Geometry: final body of the model. Coordinates: model frame, mm. A direction names the side the tool comes from. Give positions to 0.01 mm unless a question says otherwise; leave off trailing zeros. Write each loop counter-clockwise with the first axis right and the second up, starting at its lowest first coordinate (ties: lowest second). Pieces come first, ordered by that corner, then holes.
Q1. Cut plane A-A on y = 17.78. Return the cut outline in (x, z) (1 decimal), plus the area to 3 significant figures.
Q2. Reachability of faces 1 (the face through (-9.755, 36.535, 5.017)), 2 (the face through (-1.588, -1, 25)), 3 (the face through (1.588, 1, 25)) from +Z, -Z, +X, -X, +Y, -Y: full face, straight path, thin tool, end or side. Return the list, or none.
Q3. Cut plane C-C on y = -4.5. Return the cut outline in (x, z), plus the area to 3 significant figures.
Q4. Pin query (flat end, axial travel): pin 1 (6.5 mm diameter, centred on x = -9.5, z = 17.5, fed in from -Y) (3 decimals); pin 2 (3 mm diameter, centred on x = -2.5, y = -18, fed in from -Z); pin 3 (8 mm diameter, centred on x = 8.5, z = 39.5, fed in from +Y) (3 decimals). Return the tip coordinate at first contact, or that it passes through.
Q5. Line query: L1, parallel to Y at x = 0, z = 25; L2, parallel to Z at x = -0.5, y = 17.78 (3 decimals); L3, parallel to Y at x = 0, z = 18. Output: solid intervals per line, ascending.
Q6. Cut plane D-D on z = 20. Return the cut outline in (x, y) (1 decimal), plus the area to 3 significant figures.
Q7. Draft query along Y for faces 4 (the face through (-14.288, 36, 25)), 5 (the face through (-8, 34.925, 25)), 6 (the face through (-0.02, 9.25, 38.79)). Return one class per face: pulls with the +Y half, pulls with the -Y half, needs draft (parallel to the pull), parting line crosses it, or undercut.
Q8. Cut plane B-B on z = 25.4. Return the cut outline in (x, y) (1 decimal).
```python
from build123d import *

# Parameters (mm, degrees)
F0_W     = 38.1
F0_H     = 3.175
F0_W_2   = 12.7
F1_DEPTH = 50.8
F2_R     = 15.875
F3_DEPTH = 25.4
F4_R     = 1.905
F5_DEPTH = 25.4
F6_R     = 1.905
F7_DEPTH = 25.4


with BuildPart() as f1:
    # F0 (on Top) → F1 (new body)
    with BuildSketch(Plane.XY):
        with Locations((20.6375, -36.5125)):
            Rectangle(F0_W, F0_H)
        Polygon((-1.5875, -38.1), (1.5875, -38.1), (1.5875, -34.925), (1.5875, 38.1), (-1.5875, 38.1), (-1.5875, 34.925), align=None)
        with Locations((-7.9375, 36.5125)):
            Rectangle(F0_W_2, F0_H)
    extrude(amount=F1_DEPTH)

    # F2 (on face) → F3 (cut)
    with BuildSketch(Plane(origin=(-1.5875, 0, 0), x_dir=(0, -1, 0), z_dir=(-1, 0, 0))):
        with Locations((17.78, 25.4)):
            Circle(F2_R)
        with Locations((-17.78, 25.4)):
            Circle(F2_R)
    extrude(amount=-F3_DEPTH, mode=Mode.SUBTRACT)

    # F4 (on face) → F5 (cut)
    with BuildSketch(Plane.XZ.offset(38.1)):
        with Locations((33.3375, 46.355)):
            Circle(F4_R)
        with Locations((33.3375, 4.445)):
            Circle(F4_R)
    extrude(amount=-F5_DEPTH, mode=Mode.SUBTRACT)

    # F6 (on face) → F7 (cut)
    with BuildSketch(Plane(origin=(0, 38.1, 0), x_dir=(-1, 0, 0), z_dir=(0, 1, 0))):
        with Locations((7.9375, 4.445)):
            Circle(F6_R)
        with Locations((7.9375, 46.355)):
            Circle(F6_R)
    extrude(amount=-F7_DEPTH, mode=Mode.SUBTRACT)


solid = f1.part
```
Data:
1. outline: (-1.6, 0) - (1.6, 0) - (1.6, 9.5) - (-1.6, 9.5) - close; (-1.6, 41.3) - (1.6, 41.3) - (1.6, 50.8) - (-1.6, 50.8) - close
1. area: 60.5 mm2
2. face 1: +Y, -Y
2. face 2: +Z, -Z, -X, -Y
2. face 3: +Z, -Z, +X, +Y
3. outline: (-1.59, 0) - (1.59, 0) - (1.59, 16.7) - (-1.59, 16.7) - close; (-1.59, 34.1) - (1.59, 34.1) - (1.59, 50.8) - (-1.59, 50.8) - close
3. area: 106 mm2
4. pin 1: stops at y = 34.925
4. pin 2: stops at z = 0
4. pin 3: stops at y = -34.925
5. L1: y = -38.1 to -33.65, -1.91 to 1.91, 33.65 to 38.1
5. L2: z = 0 to 9.525, 41.275 to 50.8
5. L3: y = -38.1 to -31.82, -3.74 to 3.74, 31.82 to 38.1
6. outline: (-14.3, 34.9) - (-1.6, 34.9) - (-1.6, 32.7) - (1.6, 32.7) - (1.6, 38.1) - (-14.3, 38.1) - close; (-1.6, -38.1) - (39.7, -38.1) - (39.7, -34.9) - (1.6, -34.9) - (1.6, -32.7) - (-1.6, -32.7) - close; (-1.6, -2.9) - (1.6, -2.9) - (1.6, 2.9) - (-1.6, 2.9) - close
6. area: 214 mm2
7. face 4: needs draft
7. face 5: pulls with the -Y half
7. face 6: undercut
8. outline: (-14.3, 34.9) - (-1.6, 34.9) - (-1.6, 33.7) - (1.6, 33.7) - (1.6, 38.1) - (-14.3, 38.1) - close; (-1.6, -38.1) - (39.7, -38.1) - (39.7, -34.9) - (1.6, -34.9) - (1.6, -33.7) - (-1.6, -33.7) - close; (-1.6, -1.9) - (1.6, -1.9) - (1.6, 1.9) - (-1.6, 1.9) - close
